Can you work these out from the model? Positions are in its coordinate system, mm. A direction names the side the tool comes from. Give positions to 0.01 mm unless a question says otherwise; leave off trailing zeros. Order: outer loops, then holes, each group sorted by start corner. A loop starts at its lowest first (then second) coordinate and runs counter-clockwise, first axis right, second up.
Item 1: I'm going to push flat-ended pins straight in: pin 1 Ø1 at (x, y) = (3.5, 3.5) entering from +Z; pin 2 Ø2 at (x, z) = (2, 3) entering from -Y. Where does each tip first touch, or does it pass through?
Item 2: Which directions (+Z, -Z, +X, -X, +Y, -Y) give clear straight access to the entire face, cutting with the end or side of a thin tool? Please do faces 4 (the cylindrical face through (-21.19, 7.405, 4.472)), 5 (the cylindrical face through (0.56, -13.675, 1.232)).
Item 3: I want a section at D-D, the plane y = 0.5. Write out the boundary of the cut face in (x, z).
Item 4: If I drill on line 1 along Z through (x, y) = (7.5, -9); line 2 along Y through (x, z) = (-18, 1.5); line 3 along Y through (x, z) = (-7.5, 1.5), over which ranges is the centre line in solid material (lowest first)?
Item 5: I want a section at A-A, the plane x = 0. Write out the boundary of the cut face in (y, z), then the cut area to 3 significant figures.
Item 6: I want a section at B-B, the plane x = -20. Write out the boundary of the cut face in (y, z).
Item 7: If we mould it in two halves opening along Y, with no side actions, what happens to faces 1 (the cylindrical face through (-0.325, 6.853, 1.232)), 2 (the flat face through (0, 13.682, 1)), 3 (the flat face through (0, 3, 0))? For each: +Y half, -Y half, draft (parallel to the pull), parting line (faces both ways), or undercut.
Item 8: I want a section at C-C, the plane z = 3. Write out the boundary of the cut face in (x, y).
```python
from build123d import *

# Parameters (mm, degrees)
SKETCH1_R           = 1.5
BOSS_EXTRUDE1_DEPTH = 2.5
SKETCH2_R           = 1.5
BOSS_EXTRUDE2_DEPTH = 4


with BuildPart() as part:
    # Sketch1 → Boss-Extrude1 (new body)
    with BuildSketch(Plane.XY):
        with BuildLine():
            Line((-21.335922229, 13.682276209), (21.335922229, 13.682276209))
            ThreePointArc((21.335922229, 13.682276209), (0, -13.682276209), (-21.335922229, 13.682276209))
        make_face()
        with Locations((0, 8.317723791)):
            Circle(SKETCH1_R, mode=Mode.SUBTRACT)
    extrude(amount=BOSS_EXTRUDE1_DEPTH)

    # Sketch2 → Boss-Extrude2 (add)
    with BuildSketch(Plane.XY.offset(2.5)):
        with Locations((-20, 8.317723791)):
            Circle(SKETCH2_R)
    extrude(amount=BOSS_EXTRUDE2_DEPTH)


solid = part.part
```
Results list:
1. pin 1: stops at z = 2.5
1. pin 2: stops at y = -13.65
2. face 4: +Z
2. face 5: +Z, -Z
3. outline: (-20.56, 0) - (20.56, 0) - (20.56, 2.5) - (-20.56, 2.5) - close
4. line 1: z = 0 to 2.5
4. line 2: y = -4.33 to 13.68
4. line 3: y = -12.36 to 13.68
5. outline: (-13.68, 0) - (6.82, 0) - (6.82, 2.5) - (-13.68, 2.5) - close; (9.82, 0) - (13.68, 0) - (13.68, 2.5) - (9.82, 2.5) - close
5. area: 60.9 mm2
6. outline: (-0.85, 0) - (13.68, 0) - (13.68, 2.5) - (9.82, 2.5) - (9.82, 6.5) - (6.82, 6.5) - (6.82, 2.5) - (-0.85, 2.5) - close
7. face 1: undercut
7. face 2: +Y half
7. face 3: draft
8. outline: circle Ø3 at (-20, 8.32)
